Build history of the part. All positions in model axes, mm. Face numbers are marked on the shaded views. A direction names the side the tool comes from. Round coordinates to 2 decimals unless told otherwise and drop trailing zeros. Write each loop counter-clockwise with the first axis right and the second up, starting at its lowest first coordinate (ties: lowest second). Pieces come first, ordered by that corner, then holes.
Item 1: Mould opens along Y. For the marked faces 5, 6 and 7 say: +Y half, -Y half, draft (parallel to the pull), parting line (faces both ways), or undercut.
Item 2: Band-saw the part on B-B, the plane y = 37. Write the cut outline in (x, z) (3 decimals).
Item 3: Wall check: probe 1 along Z at (x, y) = (85, 10) (3 decimals); probe 2 along X at (y, z) = (51.5, 4) (3 decimals); probe 3 along Y at (x, z) = (-17, 33) (3 decimals). Give the ranges that are in metal, low to high.
Item 4: 3-axis set-ups, long thin cutter, end or side, ignore diameter. For the marked faces 1, 2, 3 and 4: which of +Z, -Z, +X, -X, +Y, -Y reach the whole face in a straight line?
Item 5: Band-saw the part on A-A, the plane x = 65.5. Write the cut outline in (y, z) (3 decimals), then the cut area to 3 significant figures.
Item 6: Drop flat-ended pins along their axis: pin 1 Ø15.5 at (x, z) = (-16.5, 30.5) entering from +Y (3 decimals); pin 2 Ø2.5 at (y, z) = (0.5, 65.5) entering from -X (3 decimals); pin 3 Ø5 at (y, z) = (16.5, 21.5) entering from -X (3 decimals); pin 4 Ø17 at (x, z) = (64.5, 24) entering from +Y. Give the stop position or say it passes through.
```python
from build123d import *

# Parameters (mm, degrees)
F1_DEPTH = 63.5
F2_DEPTH = 25.4
F3_DEPTH = 9.525


with BuildPart() as f1:
    # F0 (on Front) → F1 (new body, symmetric)
    with BuildSketch(Plane.XZ):
        Polygon((-41.275, -9.525), (41.275, -9.525), (41.275, 9.525), (22.225, 9.525), (-41.275, 9.525), align=None)
    extrude(amount=F1_DEPTH, both=True)

    # F0 (on Front) → F2 (join, symmetric)
    with BuildSketch(Plane.XZ):
        with BuildLine():
            Line((22.225, 9.525), (41.275, 9.525))
            Line((41.275, 9.525), (41.275, 27.0002))
            ThreePointArc((41.275, 27.0002), (45.92468, 38.22552), (57.15, 42.8752))
            Line((57.15, 42.8752), (60.325, 42.8752))
            Line((60.325, 42.8752), (60.325, 61.9252))
            Line((60.325, 61.9252), (57.15, 61.9252))
            add(Edge.make_bspline(
                [(55.875812, 61.901949), (56.300707, 61.910085), (56.725448, 61.917827), (57.15, 61.9252)],
                knots=[110.51738, 110.51738, 110.51738, 110.51738, 111.504536, 111.504536, 111.504536, 111.504536], degree=3))
            ThreePointArc((55.875812, 61.901949), (32.007838, 51.241225), (22.225, 27.0002))
            Line((22.225, 27.0002), (22.225, 9.525))
        make_face()
        Polygon((60.325, 61.9252), (60.325, 42.8752), (60.325, 38.1), (111.125, 38.1), (111.125, 66.675), (60.325, 66.675), align=None)
    extrude(amount=F2_DEPTH, both=True)

    # F0 (on Front) → F3 (join, symmetric)
    with BuildSketch(Plane.XZ):
        with BuildLine():
            add(Edge.make_bspline(
                [(-41.275, 9.525), (-41.187675, 55.142385), (8.306509, 60.991071), (55.875812, 61.901949)],
                knots=[0, 0, 0, 0, 110.51738, 110.51738, 110.51738, 110.51738], degree=3))
            Line((-41.275, 9.525), (22.225, 9.525))
            Line((22.225, 9.525), (22.225, 27.0002))
            ThreePointArc((22.225, 27.0002), (32.007838, 51.241225), (55.875812, 61.901949))
        make_face()
    extrude(amount=F3_DEPTH, both=True)


solid = f1.part
```
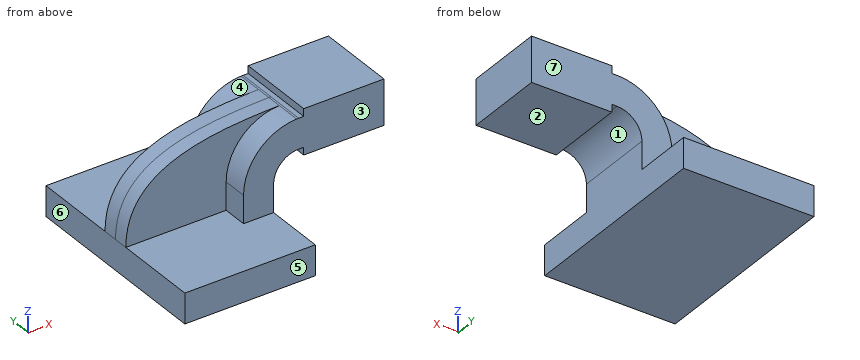
Results:
1. face 5: -Y half
1. face 6: draft
1. face 7: +Y half
2. outline: (-41.275, -9.525) - (41.275, -9.525) - (41.275, 9.525) - (-41.275, 9.525) - close
3. probe 1: z = 38.1 to 66.675
3. probe 2: x = -41.275 to 41.275
3. probe 3: y = -9.525 to 9.525
4. face 1: -Z, +Y, -Y
4. face 2: -Z, +X, +Y, -Y
4. face 3: +Z, +X, -X, -Y
4. face 4: +Z, -X, +Y
5. outline: (-25.4, 38.1) - (25.4, 38.1) - (25.4, 66.675) - (-25.4, 66.675) - close
5. area: 1,450 mm2
6. pin 1: stops at y = 9.525
6. pin 2: stops at x = 60.325
6. pin 3: stops at x = 22.225
6. pin 4: passes through
